from build123d import *

# Parameters (mm, degrees)
F0_R     = 7.5
F1_DEPTH = 20
F3_D     = 5.4
F3_DEPTH = 20
F3_TIP   = 1.6223236714
F5_D     = 6


with BuildPart() as f1:
    # F0 (on Front) → F1 (new body)
    with BuildSketch(Plane.XZ):
        with BuildLine():
            Line((-37, -39), (8.3782552843, -19.2562934749))
            ThreePointArc((8.3782552843, -19.2562934749), (20.8130885481, 2.7955938707), (3, 20.7846096908))
            Line((3, 20.7846096908), (3, 59.3))
            Line((3, 59.3), (-37, 59.3))
            Line((-37, 59.3), (-37, -39))
        make_face()
        Circle(F0_R, mode=Mode.SUBTRACT)
    extrude(amount=F1_DEPTH)

    # F3
    with Locations(Plane.XY.offset(59.3)):
        with Locations((-29, -12.5), (-5, -12.5)):
            Hole(F3_D / 2, depth=F3_DEPTH)
            with Locations((0, 0, -(F3_DEPTH + F3_TIP / 2))):  # 118° drill point
                Cone(0, F3_D / 2, F3_TIP, mode=Mode.SUBTRACT)

    # F5 (through all)
    with Locations(Plane.XZ.offset(20)):
        with Locations((-26, 32), (-26, 2)):
            Hole(F5_D / 2)


solid = f1.part
Read the model definition and answer for the solid it produces. Units are mm, in the model's axes. A direction names the side the tool comes from. Round coordinates to 2 decimals unless told otherwise and drop trailing zeros. Write each loop counter-clockwise with the first axis right and the second up, starting at its lowest first coordinate (ties: lowest second). Pieces come first, ordered by that corner, then holes. Notation, with made-up numbers: M -11,84.5 L -1,84.5 A10 ccw -1,91.5 Z; hole C 13,84 d2. An arc over 180 degrees is marked long. Use a Markdown table: item, result.
1) Flat-ended cylindrical pins translate along their axes: pin 1 (1.5 mm diameter, centred on x = 7.5, y = -17, fed in from +Z); pin 2 (3 mm diameter, centred on x = -5, y = -12.5, fed in from -Z); pin 3 (4 mm diameter, centred on x = -23, z = -10.5, fed in from +Y); pin 4 (6 mm diameter, centred on x = -29, y = -12.5, fed in from -Z). Find the tip coordinate at first contact, or state that the pin passes through.
Answers follow:
| item | result |
|---|---|
| pin 1 | stops at z = 19.89 |
| pin 2 | stops at z = -25.73 |
| pin 3 | stops at y = 0 |
| pin 4 | stops at z = -36.82 |
2) Straight lines are drawn through the part: line 1 along Z through (x, y) = (-28, -11); line 2 along X through (y, z) = (-12.5, 50); line 3 along X through (y, z) = (-10.25, 42.5). For each, find the intervals that lie inside material, in ascending order. Write a range as [from, to].
Answers follow:
| item | result |
|---|---|
| line 1 | z = [-35.08, -0.24], [4.24, 29.76], [34.24, 38.76] |
| line 2 | x = [-37, -31.7], [-26.3, -7.7], [-2.3, 3] |
| line 3 | x = [-37, -30.49], [-27.51, -6.49], [-3.51, 3] |
3) The part is cut by section A-A (z = 32). Write down the section's boundary in (x, y).
Answers follow:
| item | result |
|---|---|
| outline | M -37,-20 L -29,-20 L -29,0 L -37,0 Z; M -23,-20 L 3,-20 L 3,0 L -23,0 Z |
4) The part is cut by section B-B (y = -16.5). Write down the section's boundary in (x, z).
Answers follow:
| item | result |
|---|---|
| outline | M -37,-39 L 8.38,-19.26 A21 ccw 3,20.78 L 3,59.3 L -37,59.3 Z; hole C -26,2 d6; hole C -26,32 d6; hole C 0,0 d15 |
5) The part is cut by section D-D (z = 2). Write down the section's boundary in (x, y), plus the area to 3 significant figures.
Answers follow:
| item | result |
|---|---|
| outline | M -37,-20 L -29,-20 L -29,0 L -37,0 Z; M -23,-20 L -7.23,-20 L -7.23,0 L -23,0 Z; M 7.23,-20 L 20.9,-20 L 20.9,0 L 7.23,0 Z |
| area | 749 mm2 |
6) The part is cut by section C-C (x = 0). Write down the section's boundary in (y, z), plus the area to 3 significant figures.
Answers follow:
| item | result |
|---|---|
| outline | M -20,-22.9 L 0,-22.9 L 0,-7.5 L -20,-7.5 Z; M -20,7.5 L 0,7.5 L 0,59.3 L -20,59.3 Z |
| area | 1,340 mm2 |
7) For a pull along X with two mould halves and no side action, classify faces 1 (the flat face through (-14.629, -9.86, -29.266)), 2 (the flat face through (-17, -10, 59.3)), 3 (the cylindrical face through (-23, -10, 2)), 4 (the conical face through (-28.55, -12.36, 37.96)) as pulls with the +X half, pulls with the -X half, needs draft (parallel to the pull), parting line crosses it, or undercut.
Answers follow:
| item | result |
|---|---|
| face 1 | pulls with the +X half |
| face 2 | needs draft |
| face 3 | undercut |
| face 4 | undercut |
8) A tool of negligible diameter and unlimited length cuts with its end or side. For faces 5 (the cylindrical face through (-3.01, -10.675, 49.16)), 6 (the cylindrical face through (-7.493, -9.86, 0.33)), 7 (the flat face through (3, -10, 40)), from which of +Z, -Z, +X, -X, +Y, -Y can it reach the whole face along a straight path? Write none if from no direction.
Answers follow:
| item | result |
|---|---|
| face 5 | +Z |
| face 6 | +Y, -Y |
| face 7 | +Z, +X, +Y, -Y |
